from build123d import *

# Parameters (mm, degrees)
EXTRUDE_1_DEPTH        = 15
SKETCH_2_R             = 1.5
CUT_EXTRUDE_1_DEPTH    = 15
PATTERN_LINEAR_1_COUNT = 3
PATTERN_LINEAR_1_PITCH = 8
SKETCH_3_R             = 1.75
CUT_EXTRUDE_2_DEPTH    = 15
FILLET_1_R             = 4
FILLET_2_R             = 0.5


with BuildPart() as part:
    # Эскиз1 → Бобышка-Вытянуть1 (new body)
    with BuildSketch(Plane(origin=(0, 0, 0), x_dir=(1, 0, 0), z_dir=(0, 1, 0))):
        Polygon((-15, 25.980762114), (0, 0), (15, 0), (15, 4), (2.309401077, 4), (-11.535898385, 27.980762114), align=None)
    extrude(amount=EXTRUDE_1_DEPTH)

    # Эскиз2 → Вырез-Вытянуть1 (cut)
    with BuildSketch(Plane(origin=(3.464101615, 0, -2), x_dir=(-0.49999999999999806, 0, -0.8660254037844397), z_dir=(0.8660254037844397, 0, -0.49999999999999806))):
        with Locations((24, 7.5)):
            Circle(SKETCH_2_R)
    cut_extrude_1 = extrude(amount=-CUT_EXTRUDE_1_DEPTH, mode=Mode.SUBTRACT)

    # Линейный массив1: Вырез-Вытянуть1 ×3
    with Locations(*[Vector(0.49999999999999806, 0, 0.8660254037844397) * (i * PATTERN_LINEAR_1_PITCH) for i in range(1, PATTERN_LINEAR_1_COUNT)]):
        add(cut_extrude_1, mode=Mode.SUBTRACT)

    # Эскиз3 → Вырез-Вытянуть2 (cut)
    with BuildSketch(Plane(origin=(0, 0, -4), x_dir=(-1, 0, 0), z_dir=(0, 0, -1))):
        with Locations((-8.654700538, 7.5)):
            Circle(SKETCH_3_R)
    extrude(amount=-CUT_EXTRUDE_2_DEPTH, mode=Mode.SUBTRACT)

    # Скругление1
    fillet_1_edges = [part.edges().sort_by_distance(p)[0] for p in [
        (2.309401077, 7.5, -4),
    ]]
    fillet(fillet_1_edges, radius=FILLET_1_R)

    # Скругление2
    fillet_2_edges = [part.edges().sort_by_distance(p)[0] for p in [
        (0, 7.5, 0),
        (-15, 7.5, -25.980762114),
        (-11.535898385, 7.5, -27.980762114),
        (15, 7.5, -4),
        (15, 7.5, 0),
    ]]
    fillet(fillet_2_edges, radius=FILLET_2_R)


solid = part.part
Verification items for the finished model (mm, model axes). A direction names the side the tool comes from. Round coordinates to 2 decimals unless told otherwise and drop trailing zeros. Loops run counter-clockwise (first coordinate to the right, second up) from the corner with the lowest first, then second, coordinate; pieces in that order, holes last. Notation, with made-up numbers: (9.5, -9) - (43.5, -9) arc R14 cw to (43.5, 16) - close; hole circle Ø11 at (0.5, 69). An arc over 180 degrees is marked (long way). Write item = value, one per line.
Q1. Sectioned sample at A-A on y = 7.5. Record the boundary of the cut face in (x, z), plus the area to 3 significant figures.
Here are the results:
outline = (-14.75, -25.55) arc R0.5 ccw to (-14.57, -26.23) - (-11.97, -27.73) arc R0.5 ccw to (-11.29, -27.55) - (-9.29, -24.08) - (-12.75, -22.08) - close; (-11.25, -19.49) - (-7.79, -21.49) - (-5.29, -17.16) - (-8.75, -15.16) - close; (-7.25, -12.56) - (-3.79, -14.56) - (-1.29, -10.23) - (-4.75, -8.23) - close; (-3.25, -5.63) - (0.21, -7.63) - (1.15, -6) arc R4 cw to (4.62, -4) - (6.9, -4) - (6.9, 0) - (0.29, 0) arc R0.5 ccw to (-0.14, -0.25) - close; (10.4, -4) - (14.5, -4) arc R0.5 ccw to (15, -3.5) - (15, -0.5) arc R0.5 ccw to (14.5, 0) - (10.4, 0) - close
area = 121 mm^2
Q2. Sectioned sample at D-D on z = -4.5. Record the boundary of the cut face in (x, y), plus the area to 3 significant figures.
Here are the results:
outline = (-2.6, 0) - (2.68, 0) - (2.68, 15) - (-2.6, 15) - close
area = 79.2 mm^2
Q3. Tool access check on faces 1 (the flat face through (6, 7, 0)), 2 (the flat face through (11, 7, -4)). Record the directions out of +Z, -Z, +X, -X, +Y, -Y that give a thin tool (end or side, any length) a straight path to the whole face; none if there is none.
Here are the results:
face_1 = +Z, +X, -X, +Y, -Y
face_2 = -Z, +X, +Y, -Y
Q4. Sectioned sample at C-C on x = 11.75. Record the boundary of the cut face in (y, z).
Here are the results:
outline = (0, -4) - (15, -4) - (15, 0) - (0, 0) - close
Q5. Material ranges on L1, parallel to Z at x = 10.5, y = 2.5; L2, parallel to Z at x = -11.25, y = 10.75; L3, parallel to Y at x = -10, z = -21.25, recorded low to high.
Here are the results:
L1 = -4 to 0
L2 = -27.49 to -19.49
L3 = 0 to 6.12, 8.88 to 15
Q6. Sectioned sample at B-B on y = 1. Record the boundary of the cut face in (x, z).
Here are the results:
outline = (-14.75, -25.55) arc R0.5 ccw to (-14.57, -26.23) - (-11.97, -27.73) arc R0.5 ccw to (-11.29, -27.55) - (1.15, -6) arc R4 cw to (4.62, -4) - (14.5, -4) arc R0.5 ccw to (15, -3.5) - (15, -0.5) arc R0.5 ccw to (14.5, 0) - (0.29, 0) arc R0.5 ccw to (-0.14, -0.25) - close
Q7. Depth check by flat-ended pin: pin 1 (3 mm diameter, centred on x = 8.65, y = 7.5, fed in from +Z); pin 2 (3 mm diameter, centred on x = 8, y = 8.5, fed in from -Z); pin 3 (6 mm diameter, centred on y = 4, z = -21.5, fed in from +X). Enter the tip coordinate at first touch or a pass-through.
Here are the results:
pin_1 = through
pin_2 = -4
pin_3 = -6.06
Q8. Mould release check, pull along Z, two halves, no side actions. Record for faces 3 (the flat face through (-4.979, 5.728, -16.623)), 4 (the cylindrical face through (-6, 6, -15)), 5 (the cylindrical face through (-9.649, 6.587, -20.768)), 6 (the flat face through (-7.55, 5.73, -13.08)): +Z half, -Z half, draft (parallel to the pull), parting line (faces both ways), or undercut.
Here are the results:
face_3 = -Z half
face_4 = undercut
face_5 = undercut
face_6 = +Z half
